```python
from build123d import *

# Parameters (mm, degrees)
SKETCH1_W           = 190
SKETCH1_H           = 150
BOSS_EXTRUDE1_DEPTH = 20
CUT_EXTRUDE1_REACH  = 124.678
SKETCH2_R           = 26
SKETCH9_R           = 26
SKETCH9_R_2         = 21.1
BOSS_EXTRUDE2_DEPTH = 5


with BuildPart() as part:
    # Sketch1 → Boss-Extrude1 (new body)
    with BuildSketch(Plane(origin=(0, 0, 0), x_dir=(1, 0, 0), z_dir=(0, 1, 0))):
        Rectangle(SKETCH1_W, SKETCH1_H)
    extrude(amount=BOSS_EXTRUDE1_DEPTH)

    # Sketch2 → Cut-Extrude1 (cut, up to next)
    with BuildSketch(Plane(origin=(0, 20, 0), x_dir=(1, 0, 0), z_dir=(0, 1, 0)), mode=Mode.PRIVATE) as cut_extrude1_sk1:
        with Locations(Location((31.25, 0, 0), (0, 0, 270))):
            Circle(SKETCH2_R)
    cut_extrude1_tool1 = extrude(cut_extrude1_sk1.sketch, amount=-CUT_EXTRUDE1_REACH, mode=Mode.PRIVATE) & part.part
    # Sketch2 → Cut-Extrude1 (cut, up to next)
    with BuildSketch(Plane(origin=(0, 20, 0), x_dir=(1, 0, 0), z_dir=(0, 1, 0)), mode=Mode.PRIVATE) as cut_extrude1_sk2:
        with Locations(Location((-31.25, 0, 0), (0, 0, 270))):
            Circle(SKETCH2_R)
    cut_extrude1_tool2 = extrude(cut_extrude1_sk2.sketch, amount=-CUT_EXTRUDE1_REACH, mode=Mode.PRIVATE) & part.part
    add(cut_extrude1_tool1.solids().sort_by_distance((31.25, 20, 0))[0], mode=Mode.SUBTRACT)
    add(cut_extrude1_tool2.solids().sort_by_distance((-31.25, 20, 0))[0], mode=Mode.SUBTRACT)

    # Sketch9 → Boss-Extrude2 (add)
    # profile 1 of 2: a face of its own
    with BuildSketch(Plane(origin=(0, 20, 0), x_dir=(1, 0, 0), z_dir=(0, 1, 0))):
        with Locations(Location((-31.25, 0, 0), (0, 0, 270))):
            Circle(SKETCH9_R)
        with Locations(Location((-31.25, 0, 0), (0, 0, 270))):
            Circle(SKETCH9_R_2, mode=Mode.SUBTRACT)
    # profile 2 of 2: a face of its own
    with BuildSketch(Plane(origin=(0, 20, 0), x_dir=(1, 0, 0), z_dir=(0, 1, 0))):
        with Locations(Location((31.25, 0, 0), (0, 0, 270))):
            Circle(SKETCH9_R)
        with Locations(Location((31.25, 0, 0), (0, 0, 270))):
            Circle(SKETCH9_R_2, mode=Mode.SUBTRACT)
    extrude(amount=-BOSS_EXTRUDE2_DEPTH)


solid = part.part
```
The listing builds one solid part. Answer for the finished solid, in the listing's coordinates (mm). A direction names the side the tool comes from. Give positions to 0.01 mm unless a question says otherwise; leave off trailing zeros. Loops run counter-clockwise (first coordinate to the right, second up) from the corner with the lowest first, then second, coordinate; pieces in that order, holes last. Notation, with made-up numbers: M -27.75,65 L 11.25,65 A12 ccw 11.25,87 Z; hole C 22.5,8 d1. An arc over 180 degrees is marked long. One line per item, written item: value.
Q1. For faces 1 (the face through (-10.33, 17.54, -2.75)), 2 (the face through (-13.678, 7.605, -19.163)), determine the directions among +Z, -Z, +X, -X, +Y, -Y from which every point of the face is accessible in a straight line to the end or side of a thin tool.
Working result:
face 1: +Y, -Y
face 2: -Y
Q2. A cutting plane is placed at B-B on z = 0. Determine the outline of the cut face in (x, y).
Working result:
outline: M -95,0 L -57.25,0 L -57.25,15 L -52.35,15 L -52.35,20 L -95,20 Z; M -10.15,15 L -5.25,15 L -5.25,0 L 5.25,0 L 5.25,15 L 10.15,15 L 10.15,20 L -10.15,20 Z; M 52.35,15 L 57.25,15 L 57.25,0 L 95,0 L 95,20 L 52.35,20 Z
Q3. A cutting plane is placed at A-A on x = -31.25. Determine the outline of the cut face in (y, z).
Working result:
outline: M 0,-75 L 20,-75 L 20,-21.1 L 15,-21.1 L 15,-26 L 0,-26 Z; M 0,26 L 15,26 L 15,21.1 L 20,21.1 L 20,75 L 0,75 Z
Q4. Find the intervals of material crossed by line 1 (X direction, y = 5.5, z = 0); line 2 (Z direction, x = -31, y = 13.5); line 3 (Y direction, x = -46, z = 19), in increasing order. Write a range as from..to.
Working result:
line 1: x = -95..-57.25, -5.25..5.25, 57.25..95
line 2: z = -75..-26, 26..75
line 3: y = 15..20
Q5. Determine the mould class of faces 3 (the face through (-1, 10, -75)), 4 (the face through (95, 10, 1)), 5 (the face through (52.17, 17.54, -2.75)) for opening direction X: +X half, -X half, draft (parallel to the pull), parting line (faces both ways), or undercut.
Working result:
face 3: draft
face 4: +X half
face 5: undercut
Q6. A cutting plane is placed at C-C on y = 17. Determine the outline of the cut face in (x, z), then the cut area to 3 significant figures.
Working result:
outline: M -95,-75 L 95,-75 L 95,75 L -95,75 Z; hole C -31.25,0 d42.2; hole C 31.25,0 d42.2
area: 25,700 mm^2
Q7. Flat-ended cylindrical pins translate along their axes: P1, Ø1, axis at x = 26.5, z = 50, coming from the -Y side; P2, Ø15.5, axis at x = -29, z = 9, coming from the -Y side. Find the tip coordinate at first contact, or state that the pin passes through.
Working result:
P1: stops at y = 0
P2: passes through
Q8. A cutting plane is placed at D-D on x = 27. Determine the outline of the cut face in (y, z), then the cut area to 3 significant figures.
Working result:
outline: M 0,-75 L 20,-75 L 20,-20.67 L 15,-20.67 L 15,-25.65 L 0,-25.65 Z; M 0,25.65 L 15,25.65 L 15,20.67 L 20,20.67 L 20,75 L 0,75 Z
area: 2,020 mm^2
